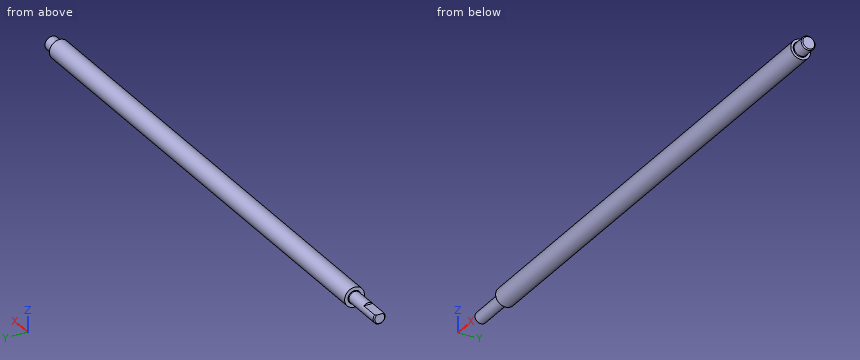
from build123d import *

# Parameters (mm, degrees)
SKETCH1_W           = 258
SKETCH1_H           = 5
SKETCH2_R           = 3
BOSS_EXTRUDE1_DEPTH = 22
CUT_EXTRUDE1_START  = -10
CUT_EXTRUDE1_DEPTH  = 10
SKETCH4_R           = 3.5
BOSS_EXTRUDE2_DEPTH = 7
CHAMFER1_SIZE       = 0.5
FILLET1_R           = 0.3


with BuildPart() as part:
    # Sketch1 → Revolve1 (revolve)
    with BuildSketch(Plane.XY, mode=Mode.PRIVATE) as revolve1_sk:
        with Locations((151, 2.5)):
            Rectangle(SKETCH1_W, SKETCH1_H)
    revolve(revolve1_sk.sketch.rotate(Axis((22, 0, 0), (1, 0, 0)), 270), axis=Axis((22, 0, 0), (1, 0, 0)))

    # Sketch2 → Boss-Extrude1 (add)
    with BuildSketch(Plane.ZY.offset(-22)):
        Circle(SKETCH2_R)
    extrude(amount=BOSS_EXTRUDE1_DEPTH)

    # Sketch3 → Cut-Extrude1 (cut)
    with BuildSketch(Plane.ZY.offset(CUT_EXTRUDE1_START)):
        with BuildLine():
            Line((2, 2.236067977), (2, -2.236067977))
            ThreePointArc((2, -2.236067977), (3, 0), (2, 2.236067977))
        make_face()
    extrude(amount=CUT_EXTRUDE1_DEPTH, mode=Mode.SUBTRACT)

    # Sketch4 → Boss-Extrude2 (add)
    with BuildSketch(Plane(origin=(280, 0, 0), x_dir=(0, 0, -1), z_dir=(1, 0, 0))):
        with Locations(Location((0, 0, 0), (0, 0, 180))):
            Circle(SKETCH4_R)
    extrude(amount=BOSS_EXTRUDE2_DEPTH)

    # Chamfer1
    chamfer1_edges = [part.edges().sort_by_distance(p)[0] for p in [
        (287, 0, -3.5),
        (0, 0, -3),
    ]]
    chamfer(chamfer1_edges, length=CHAMFER1_SIZE)

    # Fillet1
    fillet1_edges = [part.edges().sort_by_distance(p)[0] for p in [
        (280, 0, -3.5),
        (22, 0, -3),
    ]]
    fillet(fillet1_edges, radius=FILLET1_R)


solid = part.part
The listing builds one solid part. Answer for the finished solid, in the listing's coordinates (mm). Coordinates: 2 decimals unless noted, no trailing zeros. Order: outer loops, then holes, each group sorted by start corner. A loop starts at its lowest first (then second) coordinate and runs counter-clockwise, first axis right, second up.
Q1. Consider line 1 (Y direction, x = 201, z = -3.25); line 2 (X direction, y = -1, z = 3.5). Determine where each line is inside the solid, lowest interval first.
Q2. A cutting plane is placed at B-B, the plane x = 186.5. Write down the section's boundary in (y, z), and give its area (3 significant figures).
Q3. Given P1, Ø1.5, axis at x = 81, y = -3, coming from the +Z side; P2, Ø2, axis at x = 165, z = -4, coming from the -Y side; P3, Ø0.8, axis at y = 0.5, z = 2.5, coming from the -X side, each flat-ended and moving along its own axis, determine where each tip first touches the part or whether it passes through.
Q4. A cutting plane is placed at A-A, the plane z = 0. Write down the section's boundary in (x, y), and give its area (3 significant figures).
Answers follow:
1. line 1: y = -3.8 to 3.8
1. line 2: x = 22 to 280.05
2. outline: circle Ø10 at (0, 0)
2. area: 78.5 mm2
3. P1: stops at z = 4.47
3. P2: stops at y = -4
3. P3: stops at x = 10
4. outline: (0, -2.5) - (0.5, -3) - (21.7, -3) arc R0.3 cw to (22, -3.3) - (22, -5) - (280, -5) - (280, -3.8) arc R0.3 cw to (280.3, -3.5) - (286.5, -3.5) - (287, -3) - (287, 3) - (286.5, 3.5) - (280.3, 3.5) arc R0.3 cw to (280, 3.8) - (280, 5) - (22, 5) - (22, 3.3) arc R0.3 cw to (21.7, 3) - (0.5, 3) - (0, 2.5) - close
4. area: 2,760 mm2
